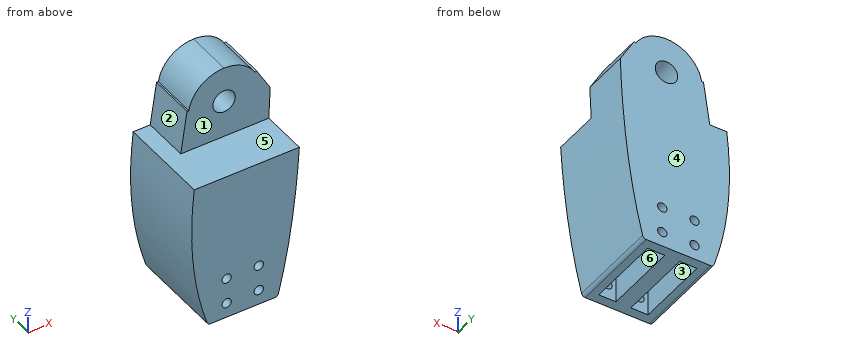
from build123d import *

# Parameters (mm, degrees)
SKETCH_1_W               = 25
SKETCH_1_H               = 25
EXTRUDE_1_DEPTH          = 59.607324229
EXTRUDE_2_DEPTH          = 25
CUT_EXTRUDE_START        = -25
CUT_EXTRUDE_4_DEPTH      = 25
SKETCH_2_R               = 3
CUT_EXTRUDE_1_DEPTH      = 36.344532851
SKETCH_4_W               = 45.98037926
SKETCH_4_H               = 12.5
CUT_EXTRUDE_2_DEPTH      = 19.5
CUT_EXTRUDE_5_DEPTH      = 17
FILLET_1_R               = 1
CUT_EXTRUDE_6_DEPTH      = 22
CUT_EXTRUDE_6_DEPTH_BACK = 20
SKETCH_8_R               = 1.25
CUT_EXTRUDE_7_DEPTH      = 10
CUT_EXTRUDE_7_DEPTH_BACK = 10
SKETCH_8_3_W             = 4.593346614
SKETCH_8_3_H             = 15


# Read off the part's stored shape, not the designer's step: the extrude step
with BuildPart() as part:
    # Sketch 1 → Extrude 1 (new body)
    with BuildSketch(Plane.XY):
        Rectangle(SKETCH_1_W, SKETCH_1_H)
    extrude(amount=EXTRUDE_1_DEPTH)

    # Sketch 6 → Extrude 2 (add)
    with BuildSketch(Plane.XZ.offset(12.5)):
        with BuildLine():
            add(Edge.make_bspline(
                [(-12.5, 59.607324229), (-21.149148663, 25.914705571), (-12.5, 0)],
                knots=[0, 0, 0, 1, 1, 1], degree=2))
            Line((-12.5, 0), (-12.5, 59.607324229))
        make_face()
    extrude(amount=-EXTRUDE_2_DEPTH)

    # Cut-Extrude 4 outline → Cut-Extrude 4 (cut)
    with BuildSketch(Plane.XZ.offset(12.5).offset(CUT_EXTRUDE_START)):
        with BuildLine():
            add(Edge.make_bspline(
                [(6.191304912, 0), (12.5, 24.95352193), (12.5, 59.607324229)],
                knots=[0, 0, 0, 1, 1, 1], degree=2))
            Line((6.191304912, 0), (12.5, 0))
            Line((12.5, 0), (12.5, 59.607324229))
        make_face()
    extrude(amount=CUT_EXTRUDE_4_DEPTH, mode=Mode.SUBTRACT)

    # Sketch 2 → Cut-Extrude 1 (cut)
    with BuildSketch(Plane(origin=(0, 12.5, 0), x_dir=(1, 0, 0), z_dir=(0, 1, 0))):
        with Locations(Location((0, -50.107324229, 0), (0, 0, 270))):
            Circle(SKETCH_2_R)
    extrude(amount=-CUT_EXTRUDE_1_DEPTH, mode=Mode.SUBTRACT)

    # Sketch 4 → Cut-Extrude 2 (cut)
    with BuildSketch(Plane.XY.offset(59.607324229)):
        with Locations((-3.730908459, -6.25)):
            Rectangle(SKETCH_4_W, SKETCH_4_H)
    extrude(amount=-CUT_EXTRUDE_2_DEPTH, mode=Mode.SUBTRACT)

    # Sketch 7 → Cut-Extrude 5 (cut)
    with BuildSketch(Plane.XZ):
        with BuildLine():
            ThreePointArc((0, 59.607324229), (4.75, 58.334565565), (8.227241336, 54.857324229))
            Line((8.227241336, 54.857324229), (8.660254038, 55.107324229))
            Line((8.660254038, 55.107324229), (12.337626898, 48.737927596))
            add(Edge.make_bspline(
                [(12.337626898, 48.737927596), (12.5, 54.047793075), (12.5, 59.607324229)],
                knots=[0, 0, 0, 1, 1, 1], degree=2))
            Line((12.5, 59.607324229), (0, 59.607324229))
        make_face()
        with BuildLine():
            Line((-9.8940238, 51.559320455), (-9.39932261, 51.486720644))
            ThreePointArc((-9.39932261, 51.486720644), (-6.21070584, 57.296005121), (0, 59.607324229))
            Line((0, 59.607324229), (-12.5, 59.607324229))
            add(Edge.make_bspline(
                [(-12.5, 59.607324229), (-15.09259901, 49.507896739), (-16.130924903, 40.107324229)],
                knots=[0, 0, 0, 1, 1, 1], degree=2))
            Line((-16.130924903, 40.107324229), (-11.574660076, 40.107324229))
            Line((-11.574660076, 40.107324229), (-9.8940238, 51.559320455))
        make_face()
    extrude(amount=-CUT_EXTRUDE_5_DEPTH, mode=Mode.SUBTRACT)

    # Fillet 1
    fillet_1_edges = [part.edges().sort_by_distance(p)[0] for p in [
        (6.191304912, 0, 0),
        (-12.5, 0, 0),
    ]]
    fillet(fillet_1_edges, radius=FILLET_1_R)

    # Sketch 8 → Cut-Extrude 6 (cut, two sides: drawn at the far end of the back side and taken through both)
    with BuildSketch(Plane(origin=(0, 0, 0), x_dir=(1, 0, 0), z_dir=(0, 1, 0)).offset(-CUT_EXTRUDE_6_DEPTH_BACK)):
        with Locations(Location((1.11398045, -4, 0), (0, 0, 270))):
            Circle(SKETCH_8_R)
        with Locations(Location((1.11398045, -11, 0), (0, 0, 270))):
            Circle(SKETCH_8_R)
        with Locations(Location((-7.479366164, -4, 0), (0, 0, 270))):
            Circle(SKETCH_8_R)
        with Locations(Location((-7.479366164, -11, 0), (0, 0, 270))):
            Circle(SKETCH_8_R)
    extrude(amount=CUT_EXTRUDE_6_DEPTH + CUT_EXTRUDE_6_DEPTH_BACK, mode=Mode.SUBTRACT)

    # Sketch 8_3 → Cut-Extrude 7 (cut, two sides: drawn at the far end of the back side and taken through both)
    with BuildSketch(Plane(origin=(0, 0, 0), x_dir=(1, 0, 0), z_dir=(0, 1, 0)).offset(-CUT_EXTRUDE_7_DEPTH_BACK)):
        with Locations((-7.479366164, -7.5)):
            Rectangle(SKETCH_8_3_W, SKETCH_8_3_H)
        with Locations((1.11398045, -7.5)):
            Rectangle(SKETCH_8_3_W, SKETCH_8_3_H)
    extrude(amount=CUT_EXTRUDE_7_DEPTH + CUT_EXTRUDE_7_DEPTH_BACK, mode=Mode.SUBTRACT)


solid = part.part
The listing builds one solid part. Answer for the finished solid, in the listing's coordinates (mm). Face numbers are marked on the shaded views. A direction names the side the tool comes from. Coordinates: 2 decimals unless noted, no trailing zeros. Write item = value, one per line. Start each with the question number.
1) The mould has two halves that part along X. Classify the marked faces 1, 2 and 3: released by +X, released by -X, zero draft, split by the parting line, or undercut.
2) A tool of negligible diameter and unlimited length cuts with its end or side. For the marked faces 4, 5 and 6, from which of +Z, -Z, +X, -X, +Y, -Y can it reach the whole face along a straight path? Write none if from no direction.
3) A cutting plane is placed at A-A (z = 11). Count the separate pieces of the cut face and the enclosed holes in it, then the cut area to 3 significant figures.
4) Straight lines are drawn through the part: line 1 (X direction, y = 10.95, z = 4); line 2 (X direction, y = -10.75, z = 11); line 3 (Z direction, x = -9.5, y = -3.5). For each, find the intervals that lie inside material, in ascending order. Write a range as from..to.
5) Given pin 1 Ø3 at (y, z) = (-7.5, 41) entering from -X; pin 2 Ø10 at (x, z) = (0.5, 53.5) entering from -Y; pin 3 Ø3 at (y, z) = (-1, 28) entering from +X, each flat-ended and moving along its own axis, determine where each tip first touches the part or whether it passes through.
Responses:
q1.face_1 = zero draft
q1.face_2 = released by -X
q1.face_3 = undercut
q2.face_4 = +Z, -Z, +X, -X, +Y
q2.face_5 = +Z, -X, -Y
q2.face_6 = -Z
q3.separate_pieces = 3
q3.enclosed_holes = 0
q3.area = 389 mm²
q4.line_1 = -13.72..-8.73, -6.23..-0.14, 2.36..7.15
q4.line_2 = -15.33..-8.73, -6.23..-0.14, 2.36..8.58
q4.line_3 = 15..40.11
q5.pin_1 = -16.2
q5.pin_2 = 0
q5.pin_3 = 11.14
